Check sheet for the drawn part. Datum: minimum x, y, z corner. Units: mm. A direction names the side the tool comes from. Give positions to 0.01 mm unless a question says otherwise; leave off trailing zeros. Order: outer loops, then holes, each group sorted by start corner. A loop starts at its lowest first (then second) coordinate and runs counter-clockwise, first axis right, second up.
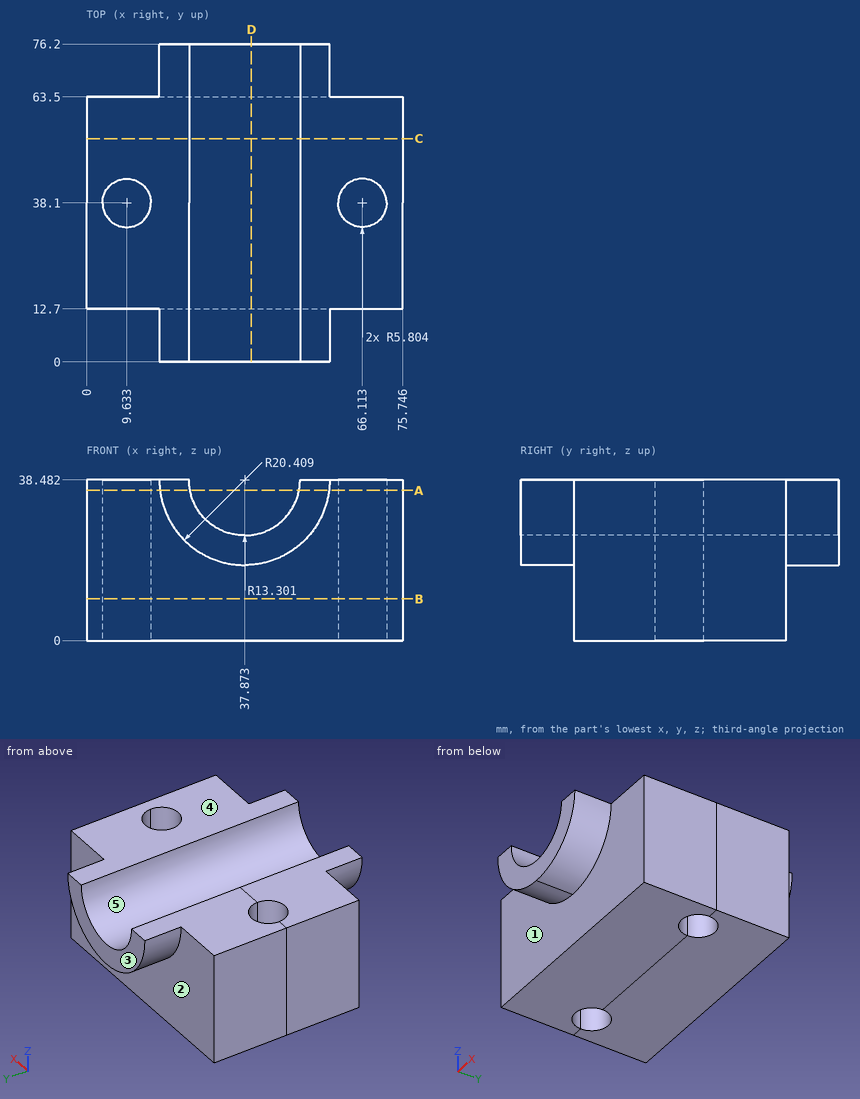
(1) Section check B-B, the plane z = 10. Enter the section's corners in (x, y) (1 decimal).
Solved:
outline: (0, 12.7) - (75.7, 12.7) - (75.7, 63.5) - (0, 63.5) - close; hole circle Ø11.6 at (9.6, 38.1); hole circle Ø11.6 at (66.1, 38.1)
(2) Go/stop test with flat-tipped pins: pin 1 (6 mm diameter, centred on x = 45, z = 6, fed in from -Y); pin 2 (5 mm diameter, centred on x = 35.5, y = 22.5, fed in from +Z) (1 decimal). Record where each tip stops, or that it passes through.
Solved:
pin 1: stops at y = 12.7
pin 2: stops at z = 26.1
(3) Set-up check for the marked faces 1, 2 and 3: record each of +Z, -Z, +X, -X, +Y, -Y from which the full face is reachable in a straight line by a thin tool's end or side.
Solved:
face 1: -Z, -Y
face 2: -Z, +Y
face 3: +Z, -Z, +X, -X, +Y
(4) Release check for a two-part mould opening along X. For the marked faces 4 and 5 record: pulls with the +X half, pulls with the -X half, needs draft (parallel to the pull), parting line crosses it, or undercut.
Solved:
face 4: needs draft
face 5: undercut
(5) Section check C-C, the plane y = 53.5. Enter the section's corners in (x, z) (1 decimal).
Solved:
outline: (0, 0) - (75.7, 0) - (75.7, 38.5) - (51.2, 38.5) arc R13.3 cw to (24.6, 38.5) - (0, 38.5) - close
(6) Section check A-A, the plane z = 36. Enter the section's corners in (x, y) (1 decimal).
Solved:
outline: (0, 12.7) - (17.6, 12.7) - (17.6, 0) - (24.8, 0) - (24.8, 76.2) - (17.6, 76.2) - (17.6, 63.5) - (0, 63.5) - close; (50.9, 0) - (58.1, 0) - (58.1, 12.7) - (75.7, 12.7) - (75.7, 63.5) - (58.1, 63.5) - (58.1, 76.2) - (50.9, 76.2) - close; hole circle Ø11.6 at (9.6, 38.1); hole circle Ø11.6 at (66.1, 38.1)
(7) Section check D-D, the plane x = 39.5. Enter the section's corners in (y, z).
Solved:
outline: (0, 18.14) - (12.7, 18.14) - (12.7, 0) - (63.5, 0) - (63.5, 18.14) - (76.2, 18.14) - (76.2, 25.28) - (0, 25.28) - close
(8) Scan lines: line 1 (X direction, y = 43, z = 20) (1 decimal); line 2 (Y direction, x = 35, z = 5); line 3 (Y direction, x = 66.5, z = 35). Record each from-to range of solid material in increasing order.
Solved:
line 1: x = 0 to 6.5, 12.7 to 63, 69.2 to 75.7
line 2: y = 12.7 to 63.5
line 3: y = 12.7 to 32.31, 43.89 to 63.5
